Could you check a few things on this drawing? It's one solid part, dimensions in mm from its lowest x, y, z. Give positions to 0.01 mm unless a question says otherwise; leave off trailing zeros. Loops run counter-clockwise (first coordinate to the right, second up) from the corner with the lowest first, then second, coordinate; pieces in that order, holes last. Notation, with made-up numbers: M 89.5,-19.5 L 106.5,-19.5 A18 cw 106.5,8.5 Z; hole C 58.25,-33.5 d8. An arc over 180 degrees is marked long. Answer as a JSON object with one key per item and string values.
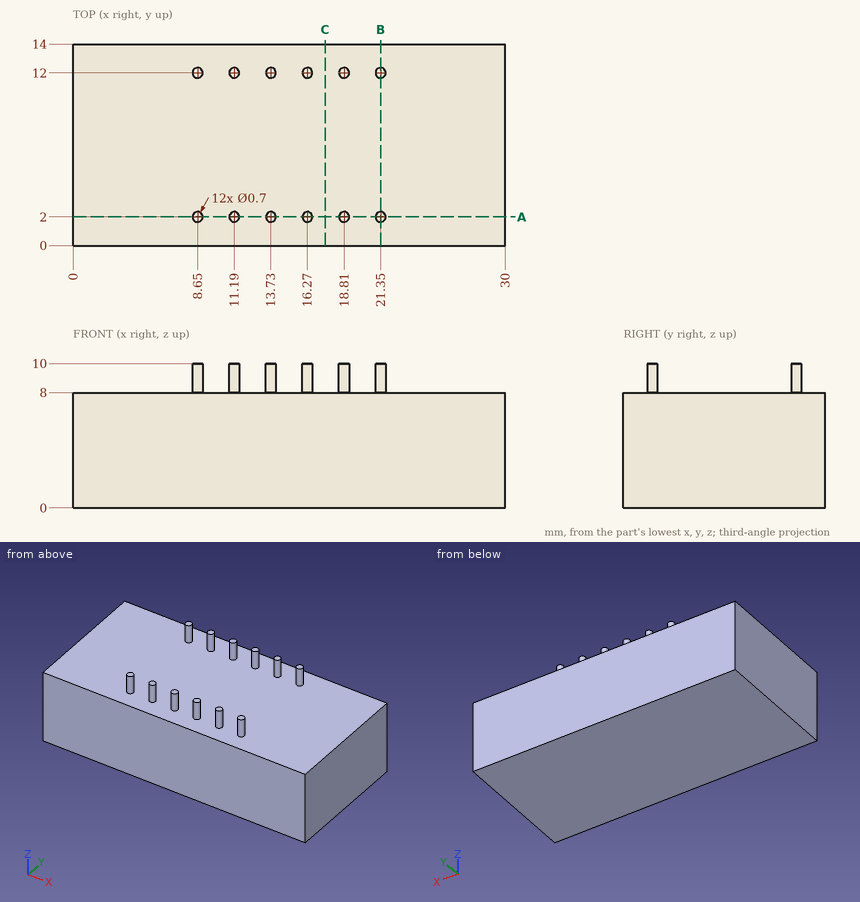
1) Suppose I cut it at B-B, the plane x = 21.35. Write out the boundary of the cut face in (y, z).
Answer list:
{"outline": "M 0,0 L 14,0 L 14,8 L 12.35,8 L 12.35,10 L 11.65,10 L 11.65,8 L 2.35,8 L 2.35,10 L 1.65,10 L 1.65,8 L 0,8 Z"}
2) Suppose I cut it at C-C, the plane x = 17.5. Write out the boundary of the cut face in (y, z), and give its area (3 significant figures).
Answer list:
{"outline": "M 0,0 L 14,0 L 14,8 L 0,8 Z", "area": "112 mm^2"}
3) Please list where these lines run through material, in increasing order: line 1 along Z through (x, y) = (15, 3.5); line 2 along Y through (x, z) = (11, 9.25). Write a range as from..to.
Answer list:
{"line 1": "0..8", "line 2": "1.71..2.29, 11.71..12.29"}
4) Suppose I cut it at A-A, the plane y = 2. Write out the boundary of the cut face in (x, z), and give its area (3 significant figures).
Answer list:
{"outline": "M 0,0 L 30,0 L 30,8 L 21.7,8 L 21.7,10 L 21,10 L 21,8 L 19.16,8 L 19.16,10 L 18.46,10 L 18.46,8 L 16.62,8 L 16.62,10 L 15.92,10 L 15.92,8 L 14.08,8 L 14.08,10 L 13.38,10 L 13.38,8 L 11.54,8 L 11.54,10 L 10.84,10 L 10.84,8 L 9,8 L 9,10 L 8.3,10 L 8.3,8 L 0,8 Z", "area": "248 mm^2"}
